Read the model definition and answer for the solid it produces. Units are mm, in the model's axes. Face numbers are marked on the shaded views. A direction names the side the tool comes from. Round coordinates to 2 decimals unless told otherwise and drop trailing zeros. Order: outer loops, then holes, each group sorted by start corner. A loop starts at its lowest first (then second) coordinate and runs counter-clockwise, first axis right, second up. Notation, with made-up numbers: (-8, 57) -> (7, 57) arc R12 ccw to (7, 62) -> close; hole circle Ø1 at (-34, -26). An arc over 180 degrees is marked (long way). One line per item, written item: value. Start each with the question number.
1. The mould has two halves that part along X. Classify the marked faces 3, 4 and 5: released by +X, released by -X, zero draft, split by the parting line, or undercut.
2. Consider line 1 (Y direction, x = 38, z = 1); line 2 (Y direction, x = 0, z = -52); line 3 (Y direction, x = 0, z = -12). Determine where each line is inside the solid, lowest interval first.
3. Section A-A (y = 38.1) is taken. Give the vertices of the cut face in (x, z).
4. Section B-B (x = 0) is taken. Give the vertices of the cut face in (y, z).
5. Section D-D (y = 0) is taken. State how many separate pieces and enclosed holes the cut face has, then the cut area to 3 significant figures.
6. For the marked faces 1 and 2, determine the directions among +Z, -Z, +X, -X, +Y, -Y from which every point of the face is accessible in a straight line to the end or side of a thin tool.
7. Flat-ended cylindrical pins translate along their axes: pin 1 Ø4 at (x, y) = (18.5, -33) entering from -Z; pin 2 Ø1.5 at (y, z) = (13.5, -8.5) entering from +X; pin 3 Ø1 at (x, z) = (-19.5, -9.5) entering from +Y; pin 4 Ø4 at (x, y) = (38.1, 38.1) entering from -Z. Find the tip coordinate at first contact, or state that the pin passes through.
8. Section C-C (x = -38.1) is taken. Give the vertices of the cut face in (y, z).
from build123d import *

# Parameters (mm, degrees)
F0_W      = 88.9
F0_H      = 88.9
F0_R      = 3.429
F1_DEPTH  = 6.35
F2_R      = 30.48
F3_DEPTH  = 6.351
F4_R      = 36.83
F4_R_2    = 30.48
F5_DEPTH  = 45.72
F6_R      = 35.56
F6_R_2    = 28.829
F7_DEPTH  = 35.56
F9_W      = 7.62
F9_H      = 7.62
F10_DEPTH = 25.49487
F11_R     = 2.794
F12_DEPTH = 44.45


with BuildPart() as f1:
    # F0 (on Top) → F1 (new body)
    with BuildSketch(Plane.XY):
        Rectangle(F0_W, F0_H)
        with Locations((-38.1, -38.1)):
            Circle(F0_R, mode=Mode.SUBTRACT)
        with Locations((38.1, -38.1)):
            Circle(F0_R, mode=Mode.SUBTRACT)
        with Locations((-38.1, 38.1)):
            Circle(F0_R, mode=Mode.SUBTRACT)
        with Locations((38.1, 38.1)):
            Circle(F0_R, mode=Mode.SUBTRACT)
    extrude(amount=F1_DEPTH)

    # F2 (on face) → F3 (cut, through all)
    with BuildSketch(Plane(origin=(0, 0, 0), x_dir=(1, 0, 0), z_dir=(0, 0, -1))):
        Circle(F2_R)
    extrude(amount=-F3_DEPTH, mode=Mode.SUBTRACT)

    # F4 (on Top) → F5 (join)
    with BuildSketch(Plane.XY):
        Circle(F4_R)
        Circle(F4_R_2, mode=Mode.SUBTRACT)
    extrude(amount=-F5_DEPTH)

    # F6 (on face) → F7 (join)
    with BuildSketch(Plane(origin=(0, 0, -45.72), x_dir=(1, 0, 0), z_dir=(0, 0, -1))):
        Circle(F6_R)
        Circle(F6_R_2, mode=Mode.SUBTRACT)
    extrude(amount=F7_DEPTH)

    # F9 (on face) → F10 (cut)
    with BuildSketch(Plane(origin=(-44.45, 0, 0), x_dir=(0, -1, 0), z_dir=(-1, 0, 0))):
        Rectangle(F9_W, F9_H)
    extrude(amount=-F10_DEPTH, mode=Mode.SUBTRACT)

    # F11 (on Right) → F12 (cut, symmetric)
    with BuildSketch(Plane.YZ):
        with Locations((0, -60.8604100329)):
            Circle(F11_R)
    extrude(amount=F12_DEPTH, both=True, mode=Mode.SUBTRACT)


solid = f1.part
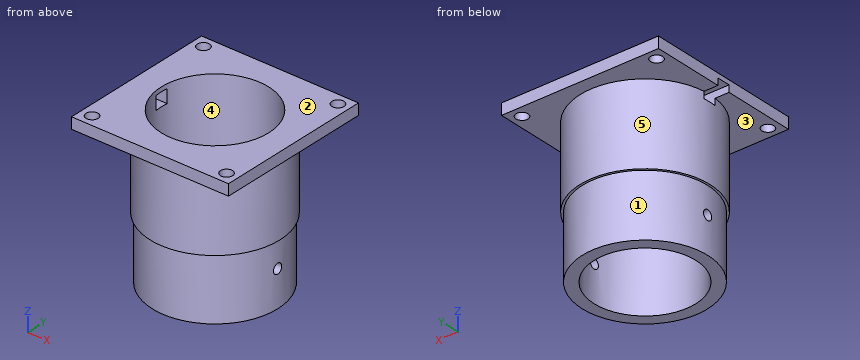
Answer:
1. face 3: zero draft
1. face 4: undercut
1. face 5: split by the parting line
2. line 1: -44.45 to -41.53, -34.67 to 34.67, 41.53 to 44.45
2. line 2: -35.56 to -28.83, 28.83 to 35.56
2. line 3: -36.83 to -30.48, 30.48 to 36.83
3. outline: (-44.45, 0) -> (-41.53, 0) -> (-41.53, 6.35) -> (-44.45, 6.35) -> close; (-34.67, 0) -> (34.67, 0) -> (34.67, 6.35) -> (-34.67, 6.35) -> close; (41.53, 0) -> (44.45, 0) -> (44.45, 6.35) -> (41.53, 6.35) -> close
4. outline: (-44.45, 0) -> (-36.83, 0) -> (-36.83, -45.72) -> (-35.56, -45.72) -> (-35.56, -81.28) -> (-28.83, -81.28) -> (-28.83, -45.72) -> (-30.48, -45.72) -> (-30.48, 6.35) -> (-44.45, 6.35) -> close; (28.83, -81.28) -> (35.56, -81.28) -> (35.56, -45.72) -> (36.83, -45.72) -> (36.83, 0) -> (44.45, 0) -> (44.45, 6.35) -> (30.48, 6.35) -> (30.48, -45.72) -> (28.83, -45.72) -> close
5. separate pieces: 5
5. enclosed holes: 0
5. area: 1,080 mm^2
6. face 1: -Z
6. face 2: +Z, +X, -X, +Y, -Y
7. pin 1: z = -45.72
7. pin 2: x = 34.55
7. pin 3: y = 31.55
7. pin 4: through
8. outline: (-44.45, 0) -> (-41.53, 0) -> (-41.53, 6.35) -> (-44.45, 6.35) -> close; (-34.67, 0) -> (-3.81, 0) -> (-3.81, 3.81) -> (3.81, 3.81) -> (3.81, 0) -> (34.67, 0) -> (34.67, 6.35) -> (-34.67, 6.35) -> close; (41.53, 0) -> (44.45, 0) -> (44.45, 6.35) -> (41.53, 6.35) -> close
